from build123d import *

# Parameters (mm, degrees)
SKETCH1_R           = 101.5
SKETCH1_R_2         = 28.956
SKETCH1_R_3         = 2.49698907
BOSS_EXTRUDE1_DEPTH = 3.175


with BuildPart() as part:
    # Sketch1 → Boss-Extrude1 (new body)
    with BuildSketch(Plane.XY):
        Circle(SKETCH1_R)
        Circle(SKETCH1_R_2, mode=Mode.SUBTRACT)
        with Locations((0, 34)):
            Circle(SKETCH1_R_3, mode=Mode.SUBTRACT)
        with Locations((17, 29.444863729)):
            Circle(SKETCH1_R_3, mode=Mode.SUBTRACT)
        with Locations((29.444863729, 17)):
            Circle(SKETCH1_R_3, mode=Mode.SUBTRACT)
        with Locations((34, 0)):
            Circle(SKETCH1_R_3, mode=Mode.SUBTRACT)
        with Locations((29.444863729, -17)):
            Circle(SKETCH1_R_3, mode=Mode.SUBTRACT)
        with Locations((17, -29.444863729)):
            Circle(SKETCH1_R_3, mode=Mode.SUBTRACT)
        with Locations((0, -34)):
            Circle(SKETCH1_R_3, mode=Mode.SUBTRACT)
        with Locations((-17, -29.444863729)):
            Circle(SKETCH1_R_3, mode=Mode.SUBTRACT)
        with Locations((-29.444863729, -17)):
            Circle(SKETCH1_R_3, mode=Mode.SUBTRACT)
        with Locations((-34, 0)):
            Circle(SKETCH1_R_3, mode=Mode.SUBTRACT)
        with Locations((-29.444863729, 17)):
            Circle(SKETCH1_R_3, mode=Mode.SUBTRACT)
        with Locations((-17, 29.444863729)):
            Circle(SKETCH1_R_3, mode=Mode.SUBTRACT)
    extrude(amount=BOSS_EXTRUDE1_DEPTH)


solid = part.part
The listing builds one solid part. Answer for the finished solid, in the listing's coordinates (mm). Coordinates: 2 decimals unless noted, no trailing zeros. Loops run counter-clockwise (first coordinate to the right, second up) from the corner with the lowest first, then second, coordinate; pieces in that order, holes last. Notation, with made-up numbers: (69, -34.5) -> (75, -34.5) arc R24 cw to (75, -14.5) -> close; hole circle Ø5 at (78.25, 1.25). An arc over 180 degrees is marked (long way). Answer in a Markdown table with one row per item. Add a question column.
1. The part is cut by section C-C, the plane z = 1.6. Count the separate pieces of the cut face and the enclosed holes in it, then the cut area to 3 significant figures.
2. Consider line 1 (Y direction, x = 0, z = 1.4); line 2 (Y direction, x = -17, z = 1.45); line 3 (X direction, y = 8.5, z = 1.75). Determine where each line is inside the solid, lowest interval first. Write a range as [from, to].
3. The part is cut by section A-A, the plane x = 0. Write down the section's boundary in (y, z) (3 decimals), then the cut area to 3 significant figures.
4. The part is cut by section D-D, the plane y = 63.5. Write down the section's boundary in (x, z) (3 decimals).
5. Flat-ended cylindrical pins translate along their axes: P1, Ø1, axis at y = -67, z = 1, coming from the -X side; P2, Ø1.5, axis at y = -50, z = 2.5, coming from the +X side. Find the tip coordinate at first contact, or state that the pin passes through.
6. The part is cut by section B-B, the plane y = -17. Write down the section's boundary in (x, z) (3 decimals), then the cut area to 3 significant figures.
7. Determine the mould class of faces 1 (the cylindrical face through (31.505, 0.11, 1.565)), 2 (the flat face through (21, -21, 0)), 3 (the cylindrical face through (96.813, 30.488, 1.565)) for opening direction X: +X half, -X half, draft (parallel to the pull), parting line (faces both ways), or undercut.
Answer below:
| question | item | result |
|---|---|---|
| 1 | separate pieces | 1 |
| 1 | enclosed holes | 13 |
| 1 | area | 29,500 mm2 |
| 2 | line 1 | [-101.5, -36.5], [-31.5, -28.96], [28.96, 31.5], [36.5, 101.5] |
| 2 | line 2 | [-100.07, -31.94], [-26.95, -23.44], [23.44, 26.95], [31.94, 100.07] |
| 2 | line 3 | [-101.14, -27.68], [27.68, 101.14] |
| 3 | outline | (-101.5, 0) -> (-36.497, 0) -> (-36.497, 3.175) -> (-101.5, 3.175) -> close; (-31.503, 0) -> (-28.956, 0) -> (-28.956, 3.175) -> (-31.503, 3.175) -> close; (28.956, 0) -> (31.503, 0) -> (31.503, 3.175) -> (28.956, 3.175) -> close; (36.497, 0) -> (101.5, 0) -> (101.5, 3.175) -> (36.497, 3.175) -> close |
| 3 | area | 429 mm2 |
| 4 | outline | (-79.183, 0) -> (79.183, 0) -> (79.183, 3.175) -> (-79.183, 3.175) -> close |
| 5 | P1 | x = -76.68 |
| 5 | P2 | x = 88.75 |
| 6 | outline | (-100.066, 0) -> (-31.942, 0) -> (-31.942, 3.175) -> (-100.066, 3.175) -> close; (-26.948, 0) -> (-23.44, 0) -> (-23.44, 3.175) -> (-26.948, 3.175) -> close; (23.44, 0) -> (26.948, 0) -> (26.948, 3.175) -> (23.44, 3.175) -> close; (31.942, 0) -> (100.066, 0) -> (100.066, 3.175) -> (31.942, 3.175) -> close |
| 6 | area | 455 mm2 |
| 7 | face 1 | undercut |
| 7 | face 2 | draft |
| 7 | face 3 | parting line |
